Input: part model. Units: mm. Frame: model coordinates. A direction names the side the tool comes from. Coordinates: 2 decimals unless noted, no trailing zeros. Order: outer loops, then holes, each group sorted by start corner. A loop starts at its lowest first (then second) coordinate and runs counter-clockwise, first axis right, second up. Notation, with made-up numbers: (60, 30.5) -> (100, 30.5) arc R15 cw to (100, 35.5) -> close; hole circle Ø8 at (7.5, -24). An arc over 180 degrees is marked (long way). Answer as CSV lines item,"result".
Autodesk Inventor part; units mm, degrees
ref_plane "YZ Plane" through (0, 0, 0) normal (1, 0, 0) x (0, 1, 0)
ref_plane "XZ Plane" through (0, 0, 0) normal (0, 1, 0) x (-1, 0, 0)
ref_plane "XY Plane" through (0, 0, 0) normal (0, 0, 1) x (1, 0, 0)
sketch "Sketch1" plane through (0, 0, 0) normal (0, 1, 0) x (-1, 0, 0)
  line L0 (193.5, 0) -> (235, 0)
  line L1 (235, 0) -> (235, 2)
  line L2 (235, 2) -> (300, 2)
  line L3 (300, 2) -> (300, 37)
  line L4 (300, 37) -> (193.5, 37)
  line L5 (193.5, 37) -> (193.5, 0)
  line L6 (0, 0) -> (0, 37)
  line L7 (0, 37) -> (193.5, 37) construction
  line L8 (0, 0) -> (193.5, 0) construction
  line L9 (-381, 381) -> (-344, 381) construction
  line L10 (-344, 381) -> (-344, 574.5) construction
  line L11 (-344, 574.5) -> (-381, 574.5)
  line L12 (-381, 574.5) -> (-381, 381) construction
  line L13 (-344, 574.5) -> (-344, 681)
  line L14 (-344, 681) -> (-379, 681)
  line L15 (-379, 681) -> (-379, 616)
  line L16 (-379, 616) -> (-381, 616)
  line L17 (-381, 616) -> (-381, 574.5)
  dimension "d0" = 387
  dimension "d1" = 600
  dimension "d2" = 470
  dimension "d3" = 2
  dimension "d4" = 37
  dimension "d6" = 2
  dimension "d7" = 37
  dimension "d8" = 387
  dimension "d9" = 470
  dimension "d10" = 600
  dimension "d11" = 381
  dimension "d12" = 381
revolve "Revolution1" add sketch "Sketch1" angle 360 about axis through (0, 0, 0) along (0, 0, 1) contours L5 L4 L3 L2 L1 L0
revolve "Revolution2" add sketch "Sketch1" angle 360 about axis through (381, 0, 381) along (-1, 0, 0) contours L11 L17 L16 L15 L14 L13
sketch "Sketch2" plane through (0, 0, 0) normal (0, 1, 0) x (-1, 0, 0)
  line L0 (-344, 574.5) -> (-344, 681)
  line L1 (300, 37) -> (193.5, 37)
  line L2 (0, 0) -> (0, 37)
  line L3 (-381, 381) -> (-344, 381)
  arc A0 (0, 37) -> (-344, 381) centre (-344, 37) ccw
sketch "Sketch3" plane through (0, 0, 37) normal (0, 0, 1) x (1, 0, 0)
  circle A0 centre (0, 0) radius 193.5
  circle A1 centre (0, 0) radius 193.5
  circle A2 centre (0, 0) radius 204.6
  dimension "d14" = 409.2
sweep "Sweep1" add profiles "Sketch3" path "Sketch2" path curves L2 A0 L3
sketch "Sketch6" plane through (0, 0, 2) normal (0, 0, -1) x (-1, 0, 0)
  circle A0 centre (0, 0) radius 300
  circle A1 centre (-52.6744, -264.812) radius 14.75
  circle A2 centre (0, 0) radius 270 construction
  line L0 (-52.6744, -264.812) -> (0, 0) construction
  line L1 (0, 0) -> (0, -270) construction
  dimension "d20" = 11.25
  dimension "d21" = 29.5
  dimension "d22" = 540
extrude "Extrusion1" cut sketch "Sketch6" against normal up to surface (35 mm away) contours A1
pattern_circular "Circular Pattern1" count 16 over 360 about axis through (0, 0, 19.5) along (0, 0, -1) of "Extrusion1"
sketch "Sketch7" plane through (379, 0, 381) normal (1, 0, 0) x (0, 0, -1)
  circle A0 centre (0, 0) radius 235
  circle A1 centre (-52.6744, -264.812) radius 14.75
  circle A2 centre (0, 0) radius 270 construction
  line L0 (-52.6744, -264.812) -> (0, 0) construction
  line L1 (0, 0) -> (0, -270) construction
  dimension "d25" = 11.25
  dimension "d26" = 29.5
  dimension "d27" = 540
extrude "Extrusion2" cut sketch "Sketch7" against normal up to surface (35 mm away) contours A1
pattern_circular "Circular Pattern2" count 16 over 360 about axis through (361.5, 0, 381) along (-1, 0, 0) of "Extrusion2"
equation "\"d0\" = d"
equation "\"d1\" = D1"
equation "\"d2\" = D2"
equation "\"d4\" = C1"
equation "\"d7\" = C1"
equation "\"d8\" = d"
equation "\"d9\" = D2"
equation "\"d10\" = D1"
equation "\"d11\" = AA"
equation "\"d12\" = AA"
equation "\"d14\" = d + 2 * t"
equation "\"d21\" = L"
equation "\"d22\" = K1"
equation "\"d26\" = L"
equation "\"d27\" = K1"
equation "\"D1\" = 600"
equation "\"C1\" = 37"
equation "\"t\" = 11.1"
equation "\"d\" = 387"
equation "\"AA\" = 381"
equation "\"D2\" = 470"
equation "\"K1\" = 540"
equation "\"L\" = 29.5"
properties part number "F90E(S)400-PN20 RF GB/T 17185-1997" material "Steel"
1. Reachability of faces 1 (the face through (-211.416, 156.819, 19.255)), 2 (the face through (228.309, 164.253, 19.255)), 3 (the face through (344, -62, 577)), 4 (the face through (361.74, 55.23, 101.66)), 5 (the face through (361.74, 148.72, 620.19)) from +Z, -Z, +X, -X, +Y, -Y: full face, straight path, thin tool, end or side. Return the list, or none.
Findings:
face 1,"+Z, -Z"
face 2,"-Z"
face 3,"none"
face 4,"+X"
face 5,"+X, -X"
2. Cut plane B-B (z = 230). State how many separate pieces and enclosed holes the cut face has, plus the area to 3 significant figures.
Findings:
separate pieces,"3"
enclosed holes,"0"
area,"23,200 mm2"
3. Mould query, pull axis X, two halves, no side actions, for faces 6 (the face through (381, 193, 415)), 7 (the face through (156.819, 211.416, 19.255)), 8 (the face through (-62, 196, 37)). Classes: released by +X, released by -X, zero draft, split by the parting line, or undercut.
Findings:
face 6,"released by +X"
face 7,"undercut"
face 8,"zero draft"
4. Contact query for flat-ended pins moving along their axis: pin 1 (2 mm diameter, centred on x = -60.5, y = 227.5, fed in from +Z); pin 2 (8 mm diameter, centred on x = -186.5, z = 99.5, fed in from +Y). Output: stop coordinate, or through.
Findings:
pin 1,"stops at z = 37"
pin 2,"stops at y = 84.87"
5. Cut plane A-A (y = 0). Return the cut outline in (x, z).
Findings:
outline,"(-300, 2) -> (-235, 2) -> (-235, 0) -> (-193.5, 0) -> (-193.5, 37) arc R537.5 cw to (344, 574.5) -> (381, 574.5) -> (381, 616) -> (379, 616) -> (379, 681) -> (344, 681) -> (344, 585.6) arc R548.6 ccw to (-204.6, 37) -> (-300, 37) -> close; (193.5, 0) -> (235, 0) -> (235, 2) -> (300, 2) -> (300, 37) -> (204.6, 37) arc R139.4 cw to (344, 176.4) -> (344, 81) -> (379, 81) -> (379, 146) -> (381, 146) -> (381, 187.5) -> (344, 187.5) arc R150.5 ccw to (193.5, 37) -> close"
6. Ray query, line 1 along X through (y, z) = (0, 9); line 2 along Z through (x, y) = (254, -127); line 3 along X through (y, z) = (143, 631). Return the intervals inside material, ascending.
Findings:
line 1,"x = -300 to -193.5, 193.5 to 300"
line 2,"z = 2 to 37, 197.01 to 213.37, 518.65 to 533.32"
line 3,"x = 344 to 379"
7. Cut plane C-C (y = -77). Return the cut outline in (x, z).
Findings:
outline,"(-289.95, 2) -> (-222.03, 2) -> (-222.03, 0) -> (-177.52, 0) -> (-177.52, 37) arc R521.52 cw to (344, 558.52) -> (381, 558.52) -> (381, 603.03) -> (379, 603.03) -> (379, 670.95) -> (344, 670.95) -> (344, 570.56) arc R533.56 ccw to (-189.56, 37) -> (-289.95, 37) -> close; (177.52, 0) -> (222.03, 0) -> (222.03, 2) -> (289.95, 2) -> (289.95, 37) -> (189.56, 37) arc R154.44 cw to (344, 191.44) -> (344, 91.05) -> (379, 91.05) -> (379, 158.97) -> (381, 158.97) -> (381, 203.48) -> (344, 203.48) arc R166.48 ccw to (177.52, 37) -> close"
